Geometry check sheet. Reference: the model listing, model coordinates, mm. Coordinates: 2 decimals unless noted, no trailing zeros. Loops run counter-clockwise (first coordinate to the right, second up) from the corner with the lowest first, then second, coordinate; pieces in that order, holes last. Notation, with made-up numbers: M 72,80 L 111,80 A17 ccw 111,111 Z; hole C -29,61.5 d8. An arc over 180 degrees is marked long. Use CSV: the item, a comma, the result in double quotes.
```python
from build123d import *

# Parameters (mm, degrees)
SKETCH_1_R      = 1.5
EXTRUDE_1_DEPTH = 2


with BuildPart() as part:
    # 草图1 → 凸台-拉伸1 (new body)
    with BuildSketch(Plane(origin=(0, 0, 0), x_dir=(0, 0, -1), z_dir=(1, 0, 0))):
        with BuildLine():
            ThreePointArc((-3, 0), (0, -3), (3, 0))
            ThreePointArc((3, 0), (2.811044981, 42.056649193), (4.390645546, 84.084048678))
            ThreePointArc((4.390645546, 84.084048678), (4.096153855, 84.569530493), (3.53773065, 84.466664204))
            ThreePointArc((3.53773065, 84.466664204), (0, 83), (-3.53773065, 84.466664204))
            ThreePointArc((-3.53773065, 84.466664204), (-4.096153855, 84.569530493), (-4.390645546, 84.084048678))
            ThreePointArc((-4.390645546, 84.084048678), (-2.811044981, 42.056649193), (-3, 0))
        make_face()
        with Locations((0, 80)):
            Circle(SKETCH_1_R, mode=Mode.SUBTRACT)
        with Locations((0, 60)):
            Circle(SKETCH_1_R, mode=Mode.SUBTRACT)
        Circle(SKETCH_1_R, mode=Mode.SUBTRACT)
    extrude(amount=EXTRUDE_1_DEPTH)


solid = part.part
```
1. Section check D-D, the plane y = 80. Record the cut outline in (x, z).
The answers:
outline,"M 0,-4.16 L 2,-4.16 L 2,-1.5 L 0,-1.5 Z; M 0,1.5 L 2,1.5 L 2,4.16 L 0,4.16 Z"
2. Section check B-B, the plane x = 0.6. Record the cut outline in (y, z), plus the area to 3 significant figures.
The answers:
outline,"M 0,-3 A1000 cw 84.08,-4.39 A0.5 ccw 84.47,-3.54 A5 cw 84.47,3.54 A0.5 ccw 84.08,4.39 A1000 cw 0,3 A3 ccw Z; hole C 0,0 d3; hole C 60,0 d3; hole C 80,0 d3"
area,"512 mm^2"
3. Release check for a two-part mould opening along Z. For faces 1 (the cylindrical face through (0.99, 42.65, 2.82)), 2 (the cylindrical face through (1, 41.5, -2.8)), 3 (the cylindrical face through (0.99, 0.07, 1.5)) record: +Z half, -Z half, draft (parallel to the pull), parting line (faces both ways), or undercut.
The answers:
face 1,"+Z half"
face 2,"-Z half"
face 3,"undercut"
4. Gauge pin test, flat ends, axial feed: P1, Ø2.5, axis at y = 80, z = 0, coming from the +X side; P2, Ø1, axis at x = 1.5, y = 48.5, coming from the +Z side. Record the tip position at first contact, or that the pin passes through.
The answers:
P1,"through"
P2,"z = 2.95"
5. Section check A-A, the plane z = 0. Record the cut outline in (x, y).
The answers:
outline,"M 0,-3 L 2,-3 L 2,-1.5 L 0,-1.5 Z; M 0,1.5 L 2,1.5 L 2,58.5 L 0,58.5 Z; M 0,61.5 L 2,61.5 L 2,78.5 L 0,78.5 Z; M 0,81.5 L 2,81.5 L 2,83 L 0,83 Z"
6. Thickness scan on line 1 (Y direction, x = 1.25, z = 0); line 2 (Y direction, x = 1.75, z = 0.5); line 3 (Z direction, x = 0.8, y = 27). Record the ranges inside material, lowest first. Write a range as [from, to].
The answers:
line 1,"[-3, -1.5], [1.5, 58.5], [61.5, 78.5], [81.5, 83]"
line 2,"[-2.96, -1.41], [1.41, 58.59], [61.41, 78.59], [81.41, 83.03]"
line 3,"[-2.68, 2.68]"
